from build123d import *

# Parameters (mm, degrees)
F0_W     = 30
F0_H     = 25
F1_DEPTH = 155
F2_R     = 5
F4_D     = 9
F4_DEPTH = 25
F4_TIP   = 2.7038727856
F6_D     = 11
F6_DEPTH = 25
F6_TIP   = 3.3047334047


with BuildPart() as f1:
    # F0 (on Front) → F1 (new body)
    with BuildSketch(Plane.XZ):
        with Locations((-15, 12.5)):
            Rectangle(F0_W, F0_H)
        Polygon((0, 25), (0, 0), (30, 0), (30, 25), (30, 189.8), (0, 189.8), align=None)
        with Locations((45, 12.5)):
            Rectangle(F0_W, F0_H)
    extrude(amount=F1_DEPTH)

    # F2
    f2_edges = [f1.edges().sort_by_distance(p)[0] for p in [
        (15, -155, 189.8),
        (0, -155, 107.4),
        (30, -155, 107.4),
        (45, -155, 25),
        (-15, -155, 25),
        (-30, -155, 12.5),
        (15, -155, 0),
        (60, -155, 12.5),
        (60, -77.5, 25),
        (60, -77.5, 0),
        (-30, -77.5, 25),
        (-30, -77.5, 0),
        (0, -77.5, 189.8),
        (30, -77.5, 189.8),
        (0, 0, 107.4),
        (30, 0, 107.4),
        (45, 0, 25),
        (15, 0, 0),
        (-15, 0, 25),
        (-30, 0, 12.5),
        (60, 0, 12.5),
        (15, 0, 189.8),
    ]]
    fillet(f2_edges, radius=F2_R)

    # F4
    with Locations(Plane.XY.offset(189.8)):
        with Locations((15, -27.5), (15, -125.5)):
            Hole(F4_D / 2, depth=F4_DEPTH)
            with Locations((0, 0, -(F4_DEPTH + F4_TIP / 2))):  # 118° drill point
                Cone(0, F4_D / 2, F4_TIP, mode=Mode.SUBTRACT)

    # F6
    with Locations(Plane.XY.offset(25)):
        with Locations((-12.5, -33), (-12.5, -124), (42.1827733517, -33), (42.1827733517, -124)):
            Hole(F6_D / 2, depth=F6_DEPTH)
            with Locations((0, 0, -(F6_DEPTH + F6_TIP / 2))):  # 118° drill point
                Cone(0, F6_D / 2, F6_TIP, mode=Mode.SUBTRACT)


solid = f1.part
Could you check a few things on this model? Use its own coordinates, in mm. A direction names the side the tool comes from. Give positions to 0.01 mm unless a question says otherwise; leave off trailing zeros. Order: outer loops, then holes, each group sorted by start corner. A loop starts at its lowest first (then second) coordinate and runs counter-clockwise, first axis right, second up. Notation, with made-up numbers: (81, 49.25) - (103, 49.25) arc R17 ccw to (103, 73.25) - close; hole circle Ø9 at (41.25, 33.5). An arc over 180 degrees is marked (long way). Return JSON: item names as keys, results as strings. Group by question number.
Q1. Suppose I cut it at C-C, the plane y = -79.5. Please give me the cut outline in (x, z), and give its area (3 significant figures).
Q2. Suppose I cut it at A-A, the plane x = -12.5. Please give me the cut outline in (y, z).
Q3. Thinking about a two-plate mould opening in Y: for faces 4 (the face through (59, -153, 13)), 5 (the face through (42.899, -118.547, 12.325)), 6 (the face through (42, -76, 25)), which applies, pulls with the +Y half, pulls with the -Y half, needs draft (parallel to the pull), parting line crosses it, or undercut?
Q4. Suppose I cut it at D-D, the plane x = 40. Please give me the cut outline in (y, z).
Q5. Will these pins go through, and if not, where does the flat tip stop? pin 1 Ø6.5 at (x, y) = (42.18, -124) entering from +Z; pin 2 Ø4 at (x, y) = (45.5, -74) entering from -Z; pin 3 Ø12.5 at (x, y) = (42.18, -33) entering from +Z; pin 4 Ø12 at (y, z) = (-110, 109) entering from +X.
Q6. Suppose I cut it at B-B, the plane z = 124.5. Please give me the cut outline in (x, y), and give its area (3 significant figures).
Q7. Please list where these lines run through material, in increasing order: line 1 along X through (y, z) = (-33, 10.5); line 2 along Y through (x, z) = (15, 181.5); line 3 along X through (y, z) = (-125.5, 176). Write a range as [from, to].
Q8. Which directions (+Z, -Z, +X, -X, +Y, -Y) give clear straight access to the entire face, cutting with the end or side of a thin tool? Please do faces 1 (the face through (40, -2, 24)), 2 (the face through (-10, -153, 24)), 3 (the face through (-13, -76, 25)).
Resolved:
{
 "1": {"outline": "(-30, 5) arc R5 ccw to (-25, 0) - (55, 0) arc R5 ccw to (60, 5) - (60, 20) arc R5 ccw to (55, 25) - (30, 25) - (30, 184.8) arc R5 ccw to (25, 189.8) - (5, 189.8) arc R5 ccw to (0, 184.8) - (0, 25) - (-25, 25) arc R5 ccw to (-30, 20) - close", "area": "7,160 mm2"},
 "2": {"outline": "(-155, 5) arc R5 ccw to (-150, 0) - (-129.5, 0) - (-129.5, 25) - (-150, 25) arc R5 ccw to (-155, 20) - close; (-118.5, 0) - (-38.5, 0) - (-38.5, 25) - (-118.5, 25) - close; (-27.5, 0) - (-5, 0) arc R5 ccw to (0, 5) - (0, 20) arc R5 ccw to (-5, 25) - (-27.5, 25) - close"},
 "3": {"face 4": "pulls with the -Y half", "face 5": "undercut", "face 6": "needs draft"},
 "4": {"outline": "(-155, 5) arc R5 ccw to (-150, 0) - (-129.05, 0) - (-129.05, 25) - (-150, 25) arc R5 ccw to (-155, 20) - close; (-118.95, 0) - (-38.05, 0) - (-38.05, 25) - (-118.95, 25) - close; (-27.95, 0) - (-5, 0) arc R5 ccw to (0, 5) - (0, 20) arc R5 ccw to (-5, 25) - (-27.95, 25) - close"},
 "5": {"pin 1": "passes through", "pin 2": "stops at z = 0", "pin 3": "stops at z = 25", "pin 4": "stops at x = 30"},
 "6": {"outline": "(0, -150) arc R5 ccw to (5, -155) - (25, -155) arc R5 ccw to (30, -150) - (30, -5) arc R5 ccw to (25, 0) - (5, 0) arc R5 ccw to (0, -5) - close", "area": "4,630 mm2"},
 "7": {"line 1": "x = [-30, -18], [-7, 36.68], [47.68, 60]", "line 2": "y = [-155, -130], [-121, -32], [-23, 0]", "line 3": "x = [0, 10.5], [19.5, 30]"},
 "8": {"face 1": "+Z, +X, +Y", "face 2": "+Z, -X, -Y", "face 3": "+Z, -X, +Y, -Y"}
}
